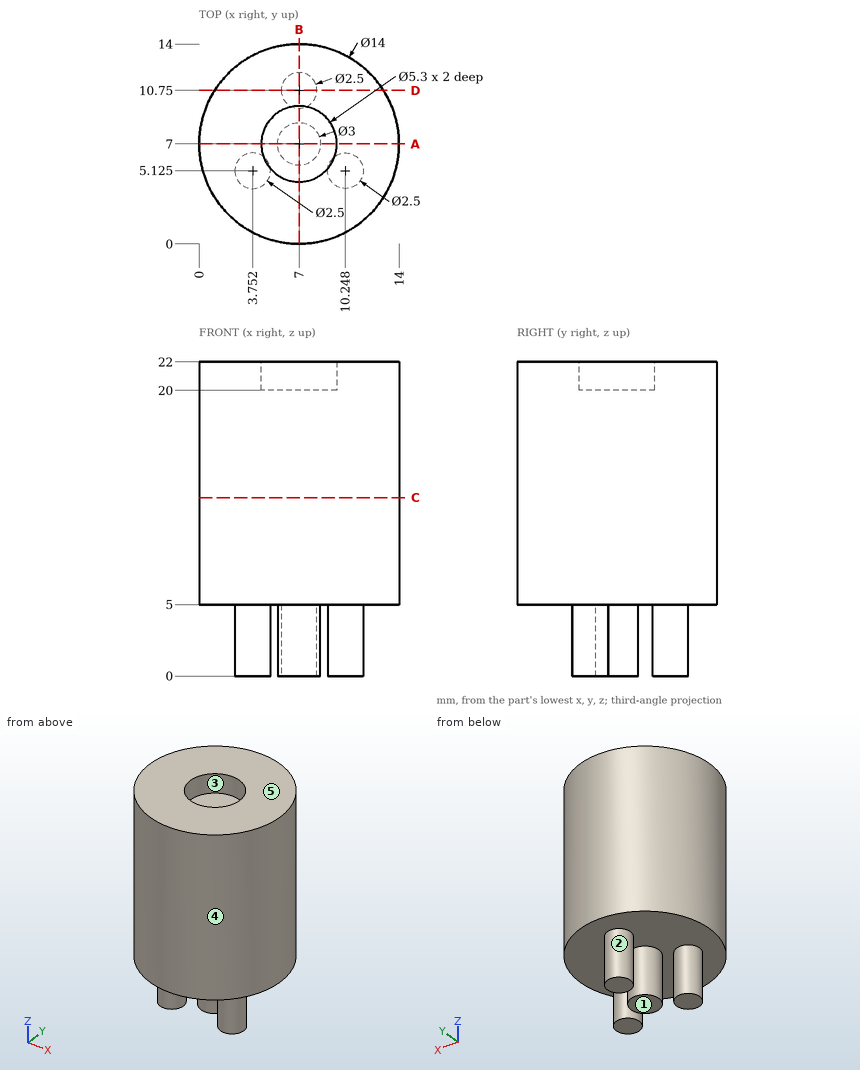
Answer from the drawing. Dimensions are ordinates in mm from the lowest x, y and z of the part. A direction names the side the tool comes from. Give positions to 0.01 mm unless a question says otherwise; leave off trailing zeros. Loops run counter-clockwise (first coordinate to the right, second up) from the corner with the lowest first, then second, coordinate; pieces in that order, holes last.
Item 1: Determine the mould class of the marked faces 3, 4 and 5 for opening direction Y: +Y half, -Y half, draft (parallel to the pull), parting line (faces both ways), or undercut.
Derived:
face 3: undercut
face 4: parting line
face 5: draft
Item 2: A cutting plane is placed at A-A (y = 7). Give the vertices of the cut face in (x, z).
Derived:
outline: (0, 5) - (5.5, 5) - (5.5, 0) - (8.5, 0) - (8.5, 5) - (14, 5) - (14, 22) - (9.65, 22) - (9.65, 20) - (4.35, 20) - (4.35, 22) - (0, 22) - close
Item 3: A tool of negligible diameter and unlimited length cuts with its end or side. For the marked faces 1 and 2, from which of +Z, -Z, +X, -X, +Y, -Y can it reach the whole face along a straight path? Write none if from no direction.
Derived:
face 1: -Z, +X, -X, +Y, -Y
face 2: -Z
Item 4: A cutting plane is placed at D-D (y = 10.75). Give the vertices of the cut face in (x, z).
Derived:
outline: (1.09, 5) - (5.75, 5) - (5.75, 0) - (8.25, 0) - (8.25, 5) - (12.91, 5) - (12.91, 22) - (1.09, 22) - close
Item 5: A cutting plane is placed at C-C (z = 12.5). Give the vertices of the cut face in (x, y), then the cut area to 3 significant figures.
Derived:
outline: circle Ø14 at (7, 7)
area: 154 mm2
Item 6: Find the intervals of material crossed by line 1 along Y through (x, z) = (7, 21.25); line 2 along X through (y, z) = (5, 2.25); line 3 along Z through (x, y) = (10.25, 1.25), in increasing order.
Derived:
line 1: y = 0 to 4.35, 9.65 to 14
line 2: x = 2.51 to 5, 9 to 11.49
line 3: z = 5 to 22
Item 7: Each of these flat-tipped pins is pushed along its axis until it touches: pin 1 Ø6 at (y, z) = (2.5, 5.5) entering from -X; pin 2 Ø2.5 at (x, y) = (6.5, 7.5) entering from +Z; pin 3 Ø1 at (x, y) = (10.5, 11) entering from -Z. Where does it stop, or does it pass through?
Derived:
pin 1: stops at x = 0.16
pin 2: stops at z = 20
pin 3: stops at z = 5
Item 8: A cutting plane is placed at B-B (x = 7). Give the vertices of the cut face in (y, z).
Derived:
outline: (0, 5) - (5.5, 5) - (5.5, 0) - (8.5, 0) - (8.5, 5) - (9.5, 5) - (9.5, 0) - (12, 0) - (12, 5) - (14, 5) - (14, 22) - (9.65, 22) - (9.65, 20) - (4.35, 20) - (4.35, 22) - (0, 22) - close
